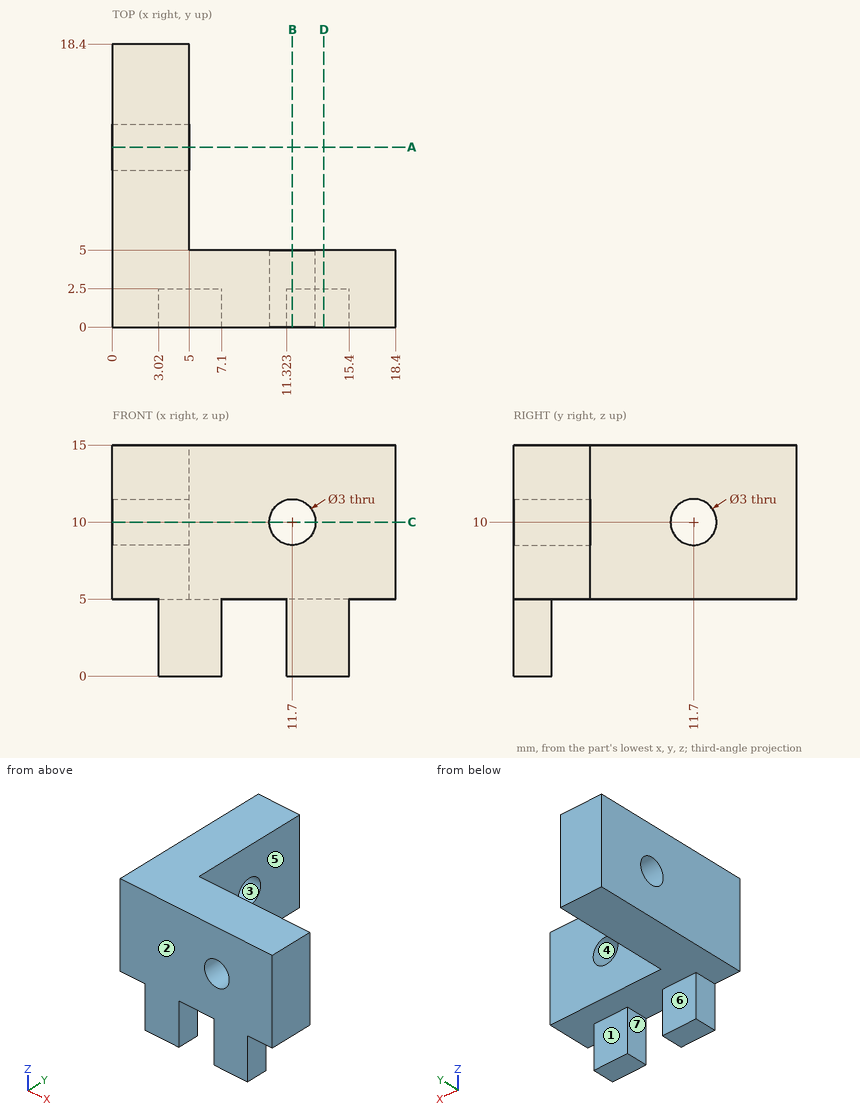
For this review, use the dimensioned drawing (mm, ordinates from the lowest corner) and the shaded views. A direction names the side the tool comes from. Round coordinates to 2 decimals unless told otherwise and drop trailing zeros. Write each loop counter-clockwise with the first axis right and the second up, starting at its lowest first coordinate (ties: lowest second). Pieces come first, ordered by that corner, then holes. Notation, with made-up numbers: (56, 11.5) -> (89, 11.5) arc R7 ccw to (89, 15.5) -> close; hole circle Ø4 at (-38, -0.75). An arc over 180 degrees is marked (long way). Answer in a Markdown table with one row per item.
Q1. For the marked faces 5, 6 and 7, list the 3-axis set-ups (+Z, -Z, +X, -X, +Y, -Y) from which the entire face can be reached by the end or side of a thin tool; tool diameter is ignored.
The answers:
| item | result |
|---|---|
| face 5 | +Z, -Z, +X, +Y |
| face 6 | -Z, +X, -X, +Y |
| face 7 | -Z, +Y, -Y |
Q2. Take a section at C-C, the plane z = 10. State the section outline as (x, y) points.
The answers:
| item | result |
|---|---|
| outline | (0, 0) -> (10.2, 0) -> (10.2, 5) -> (5, 5) -> (5, 10.2) -> (0, 10.2) -> close; (0, 13.2) -> (5, 13.2) -> (5, 18.4) -> (0, 18.4) -> close; (13.2, 0) -> (18.4, 0) -> (18.4, 5) -> (13.2, 5) -> close |
Q3. Take a section at A-A, the plane y = 11.7. State the section outline as (x, z) points, then the cut area to 3 significant figures.
The answers:
| item | result |
|---|---|
| outline | (0, 5) -> (5, 5) -> (5, 8.5) -> (0, 8.5) -> close; (0, 11.5) -> (5, 11.5) -> (5, 15) -> (0, 15) -> close |
| area | 35.0 mm² |
Q4. Clearance check with flat-ended pins moving along their axes: pin 1 Ø8 at (y, z) = (13, 12) entering from +X; pin 2 Ø5 at (x, z) = (11.7, 10) entering from +Y; pin 3 Ø2 at (y, z) = (1, 1.5) entering from +X. State where each tip first meets the part, or that it passes through.
The answers:
| item | result |
|---|---|
| pin 1 | x = 5 |
| pin 2 | y = 5 |
| pin 3 | x = 15.4 |
Q5. To check wall thickness, follow L1, parallel to Z at x = 11.7, y = 2.6; L2, parallel to Y at x = 2.1, z = 10; L3, parallel to Z at x = 11.7, y = 1.65. State the ranges of each line that lie inside material, in increasing order. Write a range as [from, to].
The answers:
| item | result |
|---|---|
| L1 | [5, 8.5], [11.5, 15] |
| L2 | [0, 10.2], [13.2, 18.4] |
| L3 | [0, 8.5], [11.5, 15] |
Q6. Take a section at B-B, the plane x = 11.7. State the section outline as (y, z) points, then the cut area to 3 significant figures.
The answers:
| item | result |
|---|---|
| outline | (0, 0) -> (2.5, 0) -> (2.5, 5) -> (5, 5) -> (5, 8.5) -> (0, 8.5) -> close; (0, 11.5) -> (5, 11.5) -> (5, 15) -> (0, 15) -> close |
| area | 47.5 mm² |
Q7. Take a section at D-D, the plane x = 13.75. State the section outline as (y, z) points, then the cut area to 3 significant figures.
The answers:
| item | result |
|---|---|
| outline | (0, 0) -> (2.5, 0) -> (2.5, 5) -> (5, 5) -> (5, 15) -> (0, 15) -> close |
| area | 62.5 mm² |
Q8. Draft analysis for pull direction Y (two halves, no side actions). For the marked faces 1, 2, 3 and 4, state which applies: +Y half, -Y half, draft (parallel to the pull), parting line (faces both ways), or undercut.
The answers:
| item | result |
|---|---|
| face 1 | +Y half |
| face 2 | -Y half |
| face 3 | undercut |
| face 4 | draft |
